Here's how the part is built. I have some questions about the finished solid (model axes, mm). Face numbers are marked on the shaded views. A direction names the side the tool comes from. Round coordinates to 2 decimals unless told otherwise and drop trailing zeros. Loops run counter-clockwise (first coordinate to the right, second up) from the corner with the lowest first, then second, coordinate; pieces in that order, holes last. Notation, with made-up numbers: (63.5, -0.5) -> (73.5, -0.5) arc R22 ccw to (73.5, 38.5) -> close; hole circle Ø3 at (53.5, 73). An arc over 180 degrees is marked (long way). Use one line per item in the form item = value. Start each with the question number.
Item 1: If we section it at C-C (z = 7.5): Write out the boundary of the cut face in (x, y).
Item 2: If I drill on L1, parallel to X at y = -0.4, z = 0; L2, parallel to X at y = -0.8, z = 0; L3, parallel to X at y = 1.45, z = 7, over which ranges is the centre line in solid material (lowest first)? Write a range as [from, to].
Item 3: Thinking about a two-plate mould opening in X: for the marked faces 1 and 2, which applies, released by +X, released by -X, zero draft, split by the parting line, or undercut?
Item 4: If we section it at D-D (y = 0.25): Write out the boundary of the cut face in (x, z).
Item 5: For the marked faces 3 and 4, which set-ups out of +Z, -Z, +X, -X, +Y, -Y let a thin tool reach every point of the face, with its end or its side?
Item 6: If we section it at B-B (z = 0.5): Write out the boundary of the cut face in (x, y).
Item 7: If we section it at A-A (x = -26): Write out the boundary of the cut face in (y, z).
Item 8: I'm going to push flat-ended pins straight in: pin 1 Ø2.5 at (x, z) = (7.25, 0) entering from +Y; pin 2 Ø2.5 at (x, z) = (1, 3.5) entering from +Y; pin 3 Ø2.5 at (x, z) = (-0.5, -2) entering from -Y; pin 4 Ø1.6 at (x, y) = (-1, 0) entering from -Z. Where does each tip first touch, or does it pass through?
```python
from build123d import *

# Parameters (mm, degrees)
SKETCH1_R             = 4.15
SKETCH1_R_2           = 1.5
BOSS_EXTRUDE1_DEPTH   = 1.5
BOSS_EXTRUDE1_2_DEPTH = 1.5
SKETCH2_W             = 8
SKETCH2_H             = 17
BOSS_EXTRUDE2_DEPTH   = 0.75


with BuildPart() as part:
    # Sketch1 → Boss-Extrude1 (new, symmetric)
    with BuildSketch(Plane(origin=(0, 0, 0), x_dir=(1, 0, 0), z_dir=(0, 1, 0))):
        Polygon((-4, -9), (-34.5, -9), (-34.5, 4), (-29.5, 9), (-4, 9), align=None)
        with Locations(Location((-26, 0, 0), (0, 0, 270))):
            Circle(SKETCH1_R, mode=Mode.SUBTRACT)
        with Locations(Location((-7.25, 0, 0), (0, 0, 270))):
            Circle(SKETCH1_R_2, mode=Mode.SUBTRACT)
    extrude(amount=BOSS_EXTRUDE1_DEPTH, both=True)



with BuildPart() as body_2:
    # Sketch1 → Boss-Extrude1 2 (new, symmetric)
    with BuildSketch(Plane(origin=(0, 0, 0), x_dir=(1, 0, 0), z_dir=(0, 1, 0))):
        Polygon((4, 9), (4, -9), (34.5, -9), (34.5, 4), (29.5, 9), align=None)
        with Locations(Location((7.25, 0, 0), (0, 0, 90))):
            Circle(SKETCH1_R_2, mode=Mode.SUBTRACT)
        with Locations(Location((26, 0, 0), (0, 0, 90))):
            Circle(SKETCH1_R, mode=Mode.SUBTRACT)
    extrude(amount=BOSS_EXTRUDE1_2_DEPTH, both=True)


with BuildPart() as part_1:
    add(part.part)

    add(body_2.part)  # Boss-Extrude2 merges body 2
    # Sketch2 → Boss-Extrude2 (add, symmetric)
    with BuildSketch(Plane(origin=(0, 0, 0), x_dir=(1, 0, 0), z_dir=(0, 1, 0))):
        Rectangle(SKETCH2_W, SKETCH2_H)
    extrude(amount=BOSS_EXTRUDE2_DEPTH, both=True)


solid = part_1.part
```
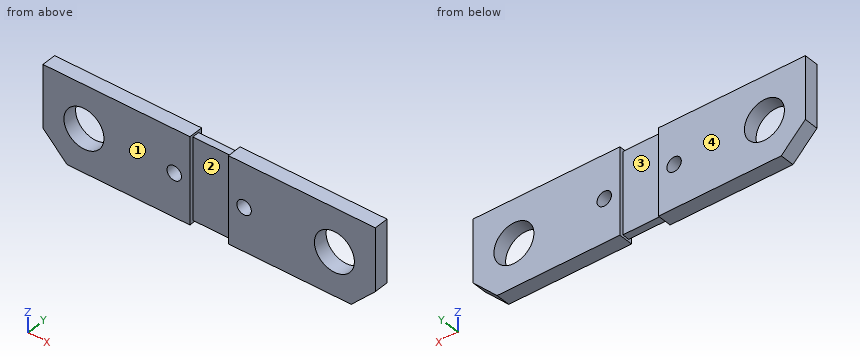
Values found:
q1.outline = (-34.5, -1.5) -> (-4, -1.5) -> (-4, -0.75) -> (4, -0.75) -> (4, -1.5) -> (34.5, -1.5) -> (34.5, 1.5) -> (4, 1.5) -> (4, 0.75) -> (-4, 0.75) -> (-4, 1.5) -> (-34.5, 1.5) -> close
q2.L1 = [-34.5, -30.15], [-21.85, -8.75], [-5.75, 5.75], [8.75, 21.85], [30.15, 34.5]
q2.L2 = [-34.5, -30.15], [-21.85, -8.75], [-5.75, -4], [4, 5.75], [8.75, 21.85], [30.15, 34.5]
q2.L3 = [-34.5, -4], [4, 34.5]
q3.face_1 = zero draft
q3.face_2 = undercut
q4.outline = (-34.5, -4) -> (-29.5, -9) -> (-4, -9) -> (-4, -8.5) -> (4, -8.5) -> (4, -9) -> (29.5, -9) -> (34.5, -4) -> (34.5, 9) -> (4, 9) -> (4, 8.5) -> (-4, 8.5) -> (-4, 9) -> (-34.5, 9) -> close; hole circle Ø8.3 at (-26, 0); hole circle Ø3 at (-7.25, 0); hole circle Ø3 at (7.25, 0); hole circle Ø8.3 at (26, 0)
q5.face_3 = +Z, -Z, +Y
q5.face_4 = +Z, -Z, +X, -X, +Y
q6.outline = (-34.5, -1.5) -> (-30.12, -1.5) -> (-30.12, 1.5) -> (-34.5, 1.5) -> close; (-21.88, -1.5) -> (-8.66, -1.5) -> (-8.66, 1.5) -> (-21.88, 1.5) -> close; (-5.84, -1.5) -> (-4, -1.5) -> (-4, -0.75) -> (4, -0.75) -> (4, -1.5) -> (5.84, -1.5) -> (5.84, 1.5) -> (4, 1.5) -> (4, 0.75) -> (-4, 0.75) -> (-4, 1.5) -> (-5.84, 1.5) -> close; (8.66, -1.5) -> (21.88, -1.5) -> (21.88, 1.5) -> (8.66, 1.5) -> close; (30.12, -1.5) -> (34.5, -1.5) -> (34.5, 1.5) -> (30.12, 1.5) -> close
q7.outline = (-1.5, -9) -> (1.5, -9) -> (1.5, -4.15) -> (-1.5, -4.15) -> close; (-1.5, 4.15) -> (1.5, 4.15) -> (1.5, 9) -> (-1.5, 9) -> close
q8.pin_1 = through
q8.pin_2 = 0.75
q8.pin_3 = -0.75
q8.pin_4 = -8.5
